Geometry check sheet. Reference: drawing and pictorial views, mm from the part's lowest x, y, z. Give positions to 0.01 mm unless a question says otherwise; leave off trailing zeros. Order: outer loops, then holes, each group sorted by start corner. A loop starts at its lowest first (then second) coordinate and runs counter-clockwise, first axis right, second up.
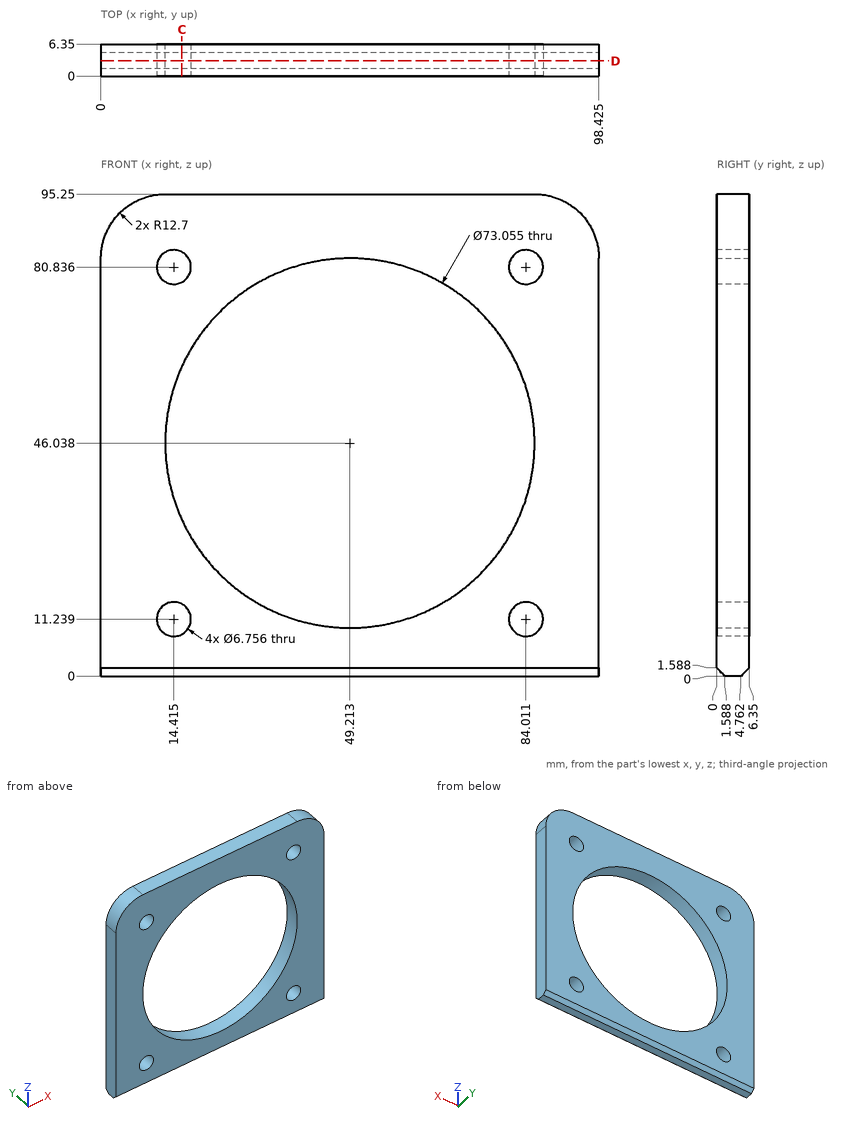
(1) Go/stop test with a flat-tipped pin: P1, Ø1, axis at y = 1.5, z = 28, coming from the -X side. Record where the tip stops, or that it passes through.
(2) Thickness scan on L1, parallel to X at y = 2.75, z = 80 (1 decimal); L2, parallel to Z at x = 37, y = 3.75; L3, parallel to X at y = 2.25, z = 72 (1 decimal). Record the ranges inside material, lowest first.
(3) Sectioned sample at C-C (x = 16). Enter the section's corners in (y, z).
(4) Sectioned sample at D-D (y = 3). Count the separate pieces of the cut face and the enclosed holes in it, plus the area to 3 significant figures.
Values follow:
1. P1: stops at x = 0
2. L1: x = 0 to 11.1, 17.7 to 35.8, 62.7 to 80.7, 87.3 to 98.4
2. L2: z = 0 to 11.61, 80.46 to 95.25
2. L3: x = 0 to 23.5, 74.9 to 98.4
3. outline: (0, 1.59) - (1.59, 0) - (4.76, 0) - (6.35, 1.59) - (6.35, 8.26) - (0, 8.26) - close; (0, 14.22) - (6.35, 14.22) - (6.35, 30.83) - (0, 30.83) - close; (0, 61.24) - (6.35, 61.24) - (6.35, 77.85) - (0, 77.85) - close; (0, 83.82) - (6.35, 83.82) - (6.35, 95.25) - (0, 95.25) - close
4. separate pieces: 1
4. enclosed holes: 5
4. area: 4,970 mm2
